Geometry: see drawing. Coordinates: mm, zero at the bounding-box minimum. A direction names the side the tool comes from. Coordinates: 2 decimals unless noted, no trailing zeros. Write each loop counter-clockwise with the first axis right and the second up, starting at its lowest first coordinate (ties: lowest second). Pieces come first, ordered by that corner, then holes.
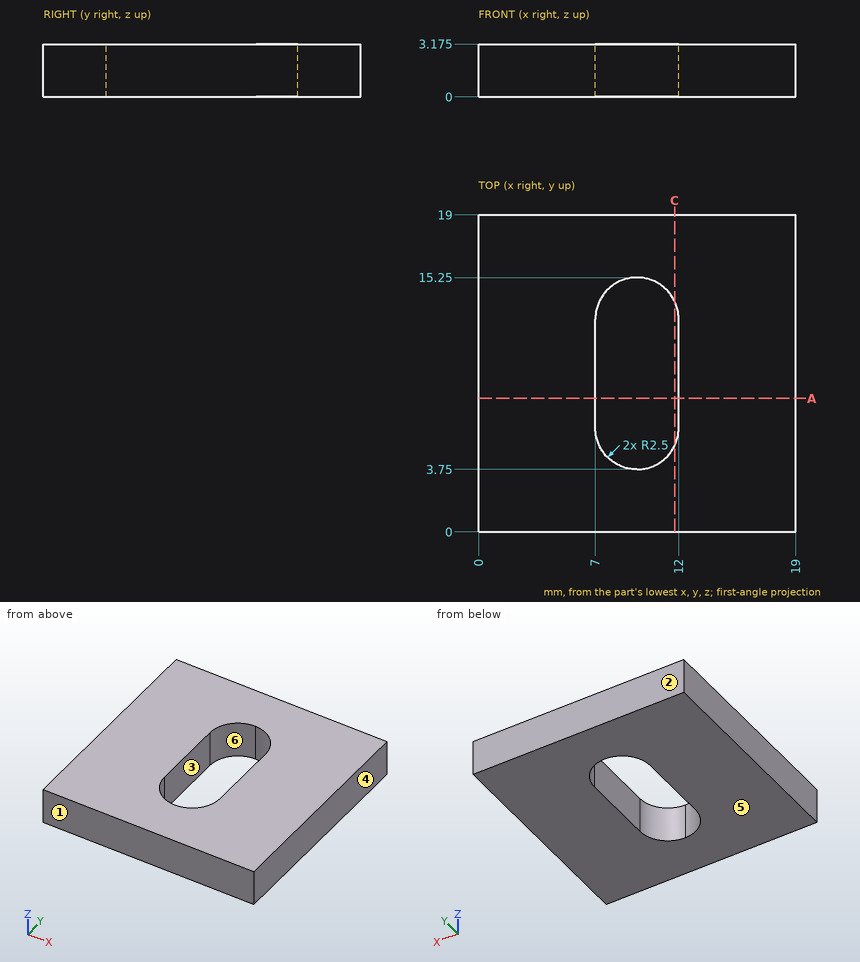
Item 1: Section A-A, the plane y = 8. Output: boundary loops of the cut face in (x, z) (3 decimals), plus the area to 4 significant figures.
Derived:
outline: (0, 0) - (7, 0) - (7, 3.175) - (0, 3.175) - close; (12, 0) - (19, 0) - (19, 3.175) - (12, 3.175) - close
area: 44.45 mm2
Item 2: Set-up query: the marked faces 5 and 6. Return all of +Z, -Z, +X, -X, +Y, -Y with unobstructed straight access to the full face (end or side cutting, diameter ignored); none if empty.
Derived:
face 5: -Z, +X, -X, +Y, -Y
face 6: +Z, -Z
Item 3: Section C-C, the plane x = 11.75. Output: boundary loops of the cut face in (y, z) (3 decimals), plus the area to 3 significant figures.
Derived:
outline: (0, 0) - (5.16, 0) - (5.16, 3.175) - (0, 3.175) - close; (13.84, 0) - (19, 0) - (19, 3.175) - (13.84, 3.175) - close
area: 32.8 mm2
Item 4: Material intervals for probe 1 along X at (y, z) = (8.5, 2.45); probe 2 along X at (y, z) = (13.75, 2); probe 3 along Y at (x, z) = (10, 2.75), sorted ascending.
Derived:
probe 1: x = 0 to 7, 12 to 19
probe 2: x = 0 to 7.21, 11.79 to 19
probe 3: y = 0 to 3.8, 15.2 to 19
Item 5: Pull-direction query (Y, two-part tool) for the marked faces 1, 2, 3 and 4; classes: released by +Y, released by -Y, zero draft, split by the parting line, or undercut.
Derived:
face 1: released by -Y
face 2: released by +Y
face 3: undercut
face 4: zero draft
